Work out the finished part from the listing and answer in its coordinate system (mm). A direction names the side the tool comes from. Give positions to 0.01 mm unless a question says otherwise; leave off trailing zeros. Order: outer loops, then holes, each group sorted by start corner. A loop starts at its lowest first (then second) coordinate and runs counter-clockwise, first axis right, second up. Notation, with made-up numbers: (6, 15.25) - (23, 15.25) arc R20 cw to (23, 35.25) - close; hole circle Ø3 at (-3.5, 74.25). An arc over 180 degrees is marked (long way). Write each question's results on one line, items separated by ' | '.
from build123d import *

# Parameters (mm, degrees)
F1_DEPTH = 152.4


with BuildPart() as f1:
    # F0 (on Top) → F1 (new body, symmetric)
    with BuildSketch(Plane.XY):
        with BuildLine():
            Line((-38.1, -50.8), (38.1, -50.8))
            ThreePointArc((38.1, -50.8), (47.0802561211, -47.0802561211), (50.8, -38.1))
            Line((50.8, -38.1), (50.8, 38.1))
            ThreePointArc((50.8, 38.1), (47.0802561211, 47.0802561211), (38.1, 50.8))
            Line((38.1, 50.8), (-38.1, 50.8))
            ThreePointArc((-38.1, 50.8), (-47.0802561211, 47.0802561211), (-50.8, 38.1))
            Line((-50.8, 38.1), (-50.8, -38.1))
            ThreePointArc((-50.8, -38.1), (-47.0802561211, -47.0802561211), (-38.1, -50.8))
        make_face()
        with BuildLine():
            ThreePointArc((38.1, 44.4499999285), (42.59012801, 42.59012801), (44.4499999285, 38.1))
            Line((44.4499999285, 38.1), (44.4499999285, -38.1))
            ThreePointArc((44.4499999285, -38.1), (42.59012801, -42.59012801), (38.1, -44.4499999285))
            Line((38.1, -44.4499999285), (-38.1, -44.4499999285))
            ThreePointArc((-38.1, -44.4499999285), (-42.59012801, -42.59012801), (-44.4499999285, -38.1))
            Line((-44.4499999285, -38.1), (-44.4499999285, 38.1))
            ThreePointArc((-44.4499999285, 38.1), (-42.59012801, 42.59012801), (-38.1, 44.4499999285))
            Line((-38.1, 44.4499999285), (38.1, 44.4499999285))
        make_face(mode=Mode.SUBTRACT)
    extrude(amount=F1_DEPTH, both=True)


solid = f1.part
1. Determine the mould class of faces 3 (the face through (-42.54, -42.64, 2.13)), 4 (the face through (-44.45, -1, 2)), 5 (the face through (0, -45, -152.4)), 6 (the face through (1, 50.8, 2)) for opening direction Y: +Y half, -Y half, draft (parallel to the pull), parting line (faces both ways), or undercut.
Answer list:
face 3: undercut | face 4: undercut | face 5: draft | face 6: +Y half
2. A tool of negligible diameter and unlimited length cuts with its end or side. For faces 1 (the face through (-1, 44.45, 2)), 2 (the face through (50.8, -1, 2)), from which of +Z, -Z, +X, -X, +Y, -Y can it reach the whole face along a straight path? Write none if from no direction.
Answer list:
face 1: +Z, -Z | face 2: +Z, -Z, +X, +Y, -Y
3. Straight lines are drawn through the part: line 1 (Y direction, x = 15, z = 73.5); line 2 (Y direction, x = -42, z = -61.5). For each, find the intervals that lie inside material, in ascending order. Write a range as [from, to].
Answer list:
line 1: [-50.8, -44.45], [44.45, 50.8] | line 2: [-50.19, -43.11], [43.11, 50.19]
4. A cutting plane is placed at B-B, the plane y = 24.5. Write down the section's boundary in (x, z).
Answer list:
outline: (-50.8, -152.4) - (-44.45, -152.4) - (-44.45, 152.4) - (-50.8, 152.4) - close; (44.45, -152.4) - (50.8, -152.4) - (50.8, 152.4) - (44.45, 152.4) - close
5. A cutting plane is placed at A-A, the plane z = 42. Write down the section's boundary in (x, y), then the cut area to 3 significant figures.
Answer list:
outline: (-50.8, -38.1) arc R12.7 ccw to (-38.1, -50.8) - (38.1, -50.8) arc R12.7 ccw to (50.8, -38.1) - (50.8, 38.1) arc R12.7 ccw to (38.1, 50.8) - (-38.1, 50.8) arc R12.7 ccw to (-50.8, 38.1) - close; hole (-44.45, -38.1) arc R6.35 ccw to (-38.1, -44.45) - (38.1, -44.45) arc R6.35 ccw to (44.45, -38.1) - (44.45, 38.1) arc R6.35 ccw to (38.1, 44.45) - (-38.1, 44.45) arc R6.35 ccw to (-44.45, 38.1) - close | area: 2,320 mm^2
